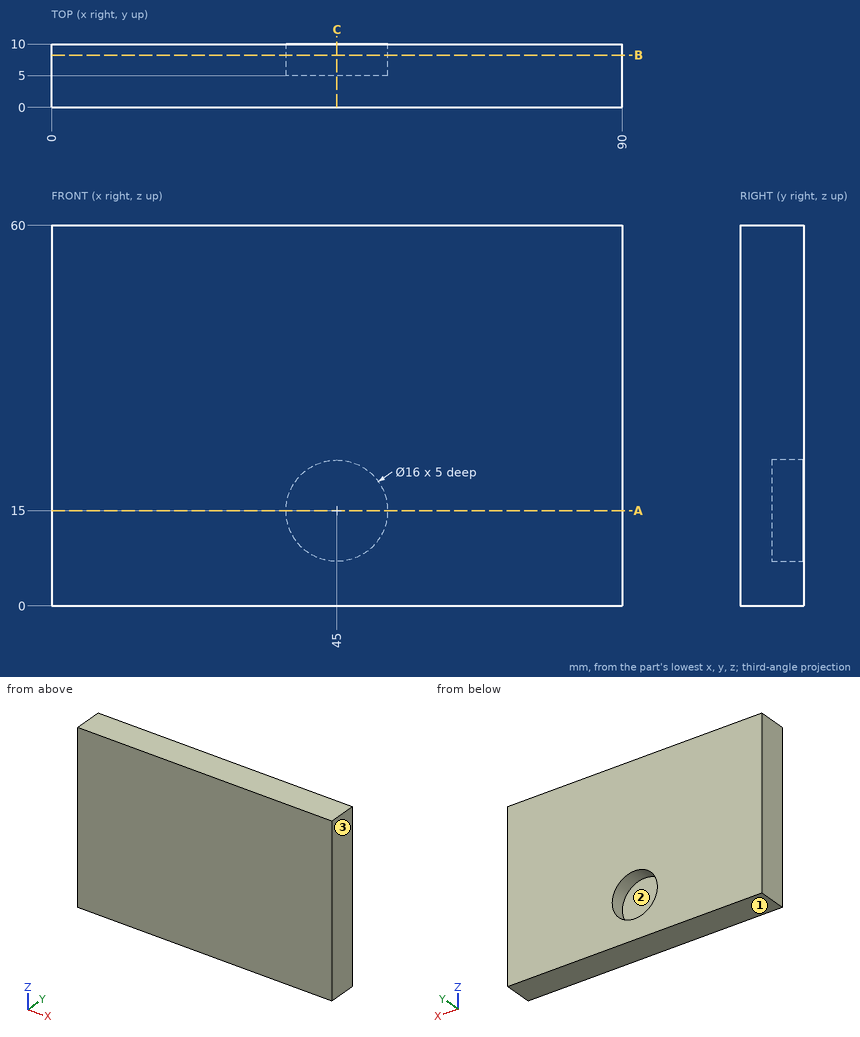
Verification items for this drawing (mm, ordinates from the low corner). Coordinates: 2 decimals unless noted, no trailing zeros. Order: outer loops, then holes, each group sorted by start corner. A loop starts at its lowest first (then second) coordinate and runs counter-clockwise, first axis right, second up. Notation, with made-up numbers: (-28.5, -20) - (28.5, -20) arc R28 cw to (28.5, 12) - close; hole circle Ø2 at (56.25, 20). An arc over 180 degrees is marked (long way). Answer in a Markdown table with one row per item. Add a question column.
1. Section check C-C (x = 45). Enter the section's corners in (y, z), plus the area to 3 significant figures.
2. Section check A-A (z = 15). Enter the section's corners in (x, y), plus the area to 3 significant figures.
3. Gauge pin test, flat end, axial feed: pin 1 Ø5 at (x, z) = (44, 17.5) entering from +Y. Record the tip position at first contact, or that the pin passes through.
4. Material ranges on L1, parallel to X at y = 6.7, z = 15; L2, parallel to Z at x = 51.5, y = 7; L3, parallel to Y at x = 42, z = 19, recorded low to high. Write a range as [from, to].
5. Section check B-B (y = 8.25). Enter the section's corners in (x, z).
6. Draft check along Z on the marked faces 1, 2 and 3. Enter one of: +Z half, -Z half, draft (parallel to the pull), parting line (faces both ways), or undercut.
Data:
| question | item | result |
|---|---|---|
| 1 | outline | (0, 0) - (10, 0) - (10, 7) - (5, 7) - (5, 23) - (10, 23) - (10, 60) - (0, 60) - close |
| 1 | area | 520 mm² |
| 2 | outline | (0, 0) - (90, 0) - (90, 10) - (53, 10) - (53, 5) - (37, 5) - (37, 10) - (0, 10) - close |
| 2 | area | 820 mm² |
| 3 | pin 1 | stops at y = 5 |
| 4 | L1 | x = [0, 37], [53, 90] |
| 4 | L2 | z = [0, 10.34], [19.66, 60] |
| 4 | L3 | y = [0, 5] |
| 5 | outline | (0, 0) - (90, 0) - (90, 60) - (0, 60) - close; hole circle Ø16 at (45, 15) |
| 6 | face 1 | -Z half |
| 6 | face 2 | undercut |
| 6 | face 3 | draft |
